from build123d import *

# Parameters (mm, degrees)
SKETCH1_R           = 11.7475
BOSS_EXTRUDE1_DEPTH = 10.795


with BuildPart() as part:
    # Sketch1 → Boss-Extrude1 (new, symmetric)
    with BuildSketch(Plane(origin=(0, 0, 0), x_dir=(1, 0, 0), z_dir=(0, 1, 0))):
        with BuildLine():
            Line((-34.925, 152.4), (34.925, 152.4))
            ThreePointArc((34.925, 152.4), (22.317119813, 76.663101875), (18.0975, 0))
            ThreePointArc((18.0975, 0), (0, -18.0975), (-18.0975, 0))
            ThreePointArc((-18.0975, 0), (-22.317119813, 76.663101875), (-34.925, 152.4))
        make_face()
        with Locations(Location((0, 0, 0), (0, 0, 270))):
            Circle(SKETCH1_R, mode=Mode.SUBTRACT)
    extrude(amount=BOSS_EXTRUDE1_DEPTH, both=True)


solid = part.part
Part model, mm, in its own coordinate system. Coordinates: 2 decimals unless noted, no trailing zeros. Loops run counter-clockwise (first coordinate to the right, second up) from the corner with the lowest first, then second, coordinate; pieces in that order, holes last. Notation, with made-up numbers: (-6.5, 25.5) - (16.5, 25.5) arc R22 cw to (16.5, 54.5) - close; hole circle Ø4 at (18.25, -7.5). An arc over 180 degrees is marked (long way). Write each question's results on one line, items separated by ' | '. Start each with the question number.
Q1. Two-plate mould, pull along Z, no slides. Class faces 1 (the flat face through (0, 10.795, -87)), 2 (the cylindrical face through (-11.468, -0.151, -2.547)), 3 (the cylindrical face through (-22.2, 0.2, -75.6)): +Z half, -Z half, draft (parallel to the pull), parting line (faces both ways), or undercut.
Q2. Drop flat-ended pins along their axis: pin 1 Ø8 at (y, z) = (-6.5, -6) entering from +X; pin 2 Ø4 at (y, z) = (6.5, -114.5) entering from +X; pin 3 Ø3 at (x, y) = (-13, -7) entering from +Z. Give the stop position or say it passes through.
Q3. Probe line 1 along Z through (x, y) = (-6, -6.25); line 2 along Z through (x, y) = (-7, -1.5); line 3 along X through (y, z) = (2.25, -137.5). List the from-to ranges inside material, lowest first.
Q4. Slice it at A-A on x = 0. Give the cut face in (y, z) (1 decimal).
Q5. Slice it at C-C on z = -34.5. Give the cut face in (x, y) (3 decimals), and give its area (3 significant figures).
Q6. Slice it at D-D on x = -22. Give the cut face in (y, z) (3 decimals).
Q7. Slice it at B-B on y = 9. Give the cut face in (x, z) (1 decimal), and give its area (3 significant figures).
Answer:
1) face 1: draft | face 2: undercut | face 3: +Z half
2) pin 1: stops at x = 18.17 | pin 2: stops at x = 27.88 | pin 3: stops at z = 13.97
3) line 1: z = -152.4 to -10.1, 10.1 to 17.07 | line 2: z = -152.4 to -9.43, 9.43 to 16.69 | line 3: x = -31.76 to 31.76
4) outline: (-10.8, -152.4) - (10.8, -152.4) - (10.8, -11.7) - (-10.8, -11.7) - close; (-10.8, 11.7) - (10.8, 11.7) - (10.8, 18.1) - (-10.8, 18.1) - close
5) outline: (-18.95, -10.795) - (18.95, -10.795) - (18.95, 10.795) - (-18.95, 10.795) - close | area: 818 mm2
6) outline: (-10.795, -152.4) - (10.795, -152.4) - (10.795, -73.734) - (-10.795, -73.734) - close
7) outline: (-34.9, -152.4) - (34.9, -152.4) arc R698.5 cw to (18.1, 0) arc R18.1 ccw to (-18.1, 0) arc R698.5 cw to start; hole circle Ø23.5 at (0, 0) | area: 7,300 mm2
